Answer from the drawing. Dimensions are ordinates in mm from the lowest x, y and z of the part. A direction names the side the tool comes from. Round coordinates to 2 decimals unless told otherwise and drop trailing zeros. Order: outer loops, then holes, each group sorted by start corner. A loop starts at its lowest first (then second) coordinate and runs counter-clockwise, first axis right, second up. Notation, with made-up numbers: (46.25, -20.75) -> (99.25, -20.75) arc R13 ccw to (99.25, -2.75) -> close; hole circle Ø1 at (-16.5, 9.25). An arc over 180 degrees is marked (long way). Use a Markdown table: item, result. Add a question column.
Item 1: Flat-ended cylindrical pins translate along their axes: P1, Ø2, axis at x = 16, y = 33.5, coming from the +Z side; P2, Ø2.5, axis at x = 11, y = 20.5, coming from the -Z side. Find the tip coordinate at first contact, or state that the pin passes through.
Item 2: A cutting plane is placed at D-D, the plane y = 18. Determine the outline of the cut face in (x, z).
Item 3: For a pull along Y with two mould halves and no side action, classify the marked faces 4, 5, 6 and 7 as +Y half, -Y half, draft (parallel to the pull), parting line (faces both ways), or undercut.
Item 4: A tool of negligible diameter and unlimited length cuts with its end or side. For the marked faces 1, 2 and 3, from which of +Z, -Z, +X, -X, +Y, -Y can it reach the whole face along a straight path? Write none if from no direction.
Item 5: A cutting plane is placed at C-C, the plane z = 1.3. Determine the outline of the cut face in (x, y), plus the area to 3 significant figures.
Item 6: A cutting plane is placed at A-A, the plane y = 36. Determine the outline of the cut face in (x, z).
Item 7: Find the intervals of material crossed by L1, parallel to X at y = 38, z = 3.95; L2, parallel to Y at x = 34.5, z = 2.3; L3, parallel to Y at x = 18.5, z = 4.5, in increasing order. Write a range as [from, to].
Item 8: A cutting plane is placed at B-B, the plane x = 27. Determine the outline of the cut face in (y, z).
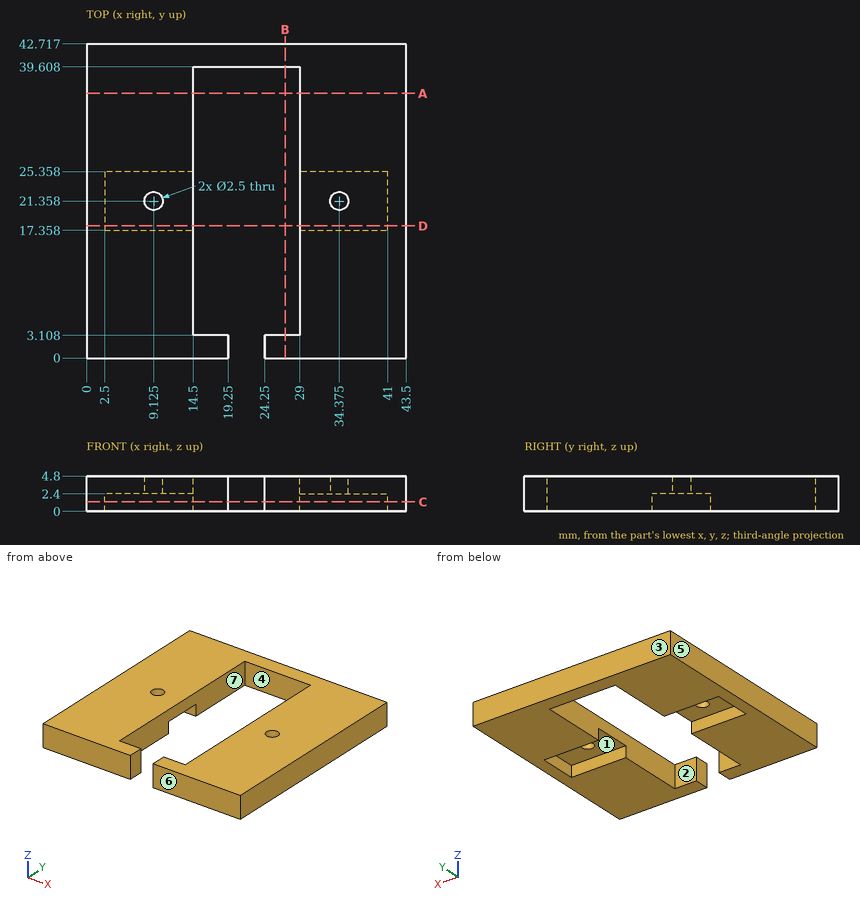
Reported:
| question | item | result |
|---|---|---|
| 1 | P1 | through |
| 1 | P2 | z = 2.4 |
| 2 | outline | (0, 0) -> (2.5, 0) -> (2.5, 2.4) -> (14.5, 2.4) -> (14.5, 4.8) -> (0, 4.8) -> close; (29, 2.4) -> (41, 2.4) -> (41, 0) -> (43.5, 0) -> (43.5, 4.8) -> (29, 4.8) -> close |
| 3 | face 4 | undercut |
| 3 | face 5 | draft |
| 3 | face 6 | -Y half |
| 3 | face 7 | undercut |
| 4 | face 1 | -Z |
| 4 | face 2 | +Z, -Z |
| 4 | face 3 | +Z, -Z, +X, -X, +Y |
| 5 | outline | (0, 0) -> (19.25, 0) -> (19.25, 3.11) -> (14.5, 3.11) -> (14.5, 17.36) -> (2.5, 17.36) -> (2.5, 25.36) -> (14.5, 25.36) -> (14.5, 39.61) -> (29, 39.61) -> (29, 25.36) -> (41, 25.36) -> (41, 17.36) -> (29, 17.36) -> (29, 3.11) -> (24.25, 3.11) -> (24.25, 0) -> (43.5, 0) -> (43.5, 42.72) -> (0, 42.72) -> close |
| 5 | area | 1,120 mm² |
| 6 | outline | (0, 0) -> (14.5, 0) -> (14.5, 4.8) -> (0, 4.8) -> close; (29, 0) -> (43.5, 0) -> (43.5, 4.8) -> (29, 4.8) -> close |
| 7 | L1 | [0, 14.5], [29, 43.5] |
| 7 | L2 | [0, 17.36], [25.36, 42.72] |
| 7 | L3 | [0, 3.11], [39.61, 42.72] |
| 8 | outline | (0, 0) -> (3.11, 0) -> (3.11, 4.8) -> (0, 4.8) -> close; (39.61, 0) -> (42.72, 0) -> (42.72, 4.8) -> (39.61, 4.8) -> close |
